Can you work these out from the model? Positions are in its coordinate system, mm. A direction names the side the tool comes from. Round coordinates to 2 decimals unless told otherwise and drop trailing zeros. Order: outer loops, then holes, each group sorted by start corner. A loop starts at its lowest first (then second) coordinate and runs counter-clockwise, first axis right, second up. Notation, with made-up numbers: (74.25, 66) -> (93.25, 66) arc R23 cw to (93.25, 80) -> close; hole circle Ø3 at (7.5, 60.25). An arc over 180 degrees is marked (long way). One line per item, written item: value.
Autodesk Inventor part; units mm, degrees
ref_plane "YZ Plane" through (0, 0, 0) normal (1, 0, 0) x (0, 1, 0)
ref_plane "XZ Plane" through (0, 0, 0) normal (0, 1, 0) x (-1, 0, 0)
ref_plane "XY Plane" through (0, 0, 0) normal (0, 0, 1) x (1, 0, 0)
sketch "Sketch1" plane through (0, 0, 0) normal (0, 1, 0) x (-1, 0, 0)
  line L0 (0, 0) -> (180.34, 0)
  line L1 (180.34, 0) -> (180.34, -76.2)
  line L2 (180.34, -76.2) -> (0, -76.2)
  line L3 (0, -76.2) -> (0, 0)
  dimension "d0" = 180.34
  dimension "d1" = 76.2
extrude "Extrusion1" add sketch "Sketch1" along normal blind 167.64
fillet "Fillet1" radius 3.175 8 edges at (-90.17, 167.64, 0) (-180.34, 167.64, -38.1) (-90.17, 167.64, -76.2) (0, 167.64, -38.1) (-90.17, 0, -76.2) (-180.34, 0, -38.1) (-90.17, 0, 0) (0, 0, -38.1)
sketch "Sketch2" plane through (0, 3.175, -76.2) normal (1, 0, 0) x (0, 0, -1)
  line L0 (0, 164.465) -> (-19.05, 164.465)
  line L1 (-19.05, 164.465) -> (-19.05, 145.415)
  line L2 (-19.05, 145.415) -> (0, 145.415)
  line L3 (0, 145.415) -> (0, 164.465)
  line L4 (0, 164.465) -> (-19.05, 164.465)
  line L5 (-19.05, 164.465) -> (-19.05, 145.415)
  line L6 (-19.05, 145.415) -> (0, 145.415)
  line L7 (0, 145.415) -> (0, 164.465)
  point P0 (-76.2, -3.175)
  dimension "d5" = 19.05
  dimension "d6" = 19.05
extrude "Extrusion2" cut sketch "Sketch2" against normal blind 50.8
sketch "Sketch3" plane through (-180.34, 3.175, 0) normal (-1, 0, 0) x (0, 0, 1)
  line L0 (-76.2, 164.465) -> (-57.15, 164.465)
  line L1 (-57.15, 164.465) -> (-57.15, 145.415)
  line L2 (-57.15, 145.415) -> (-76.2, 145.415)
  line L3 (-76.2, 145.415) -> (-76.2, 164.465)
  point P0 (0, -3.175)
  dimension "d9" = 19.05
  dimension "d10" = 19.05
extrude "Extrusion3" cut sketch "Sketch3" against normal blind 50.8
fillet "Fillet2" radius 3.175 22 edges at (-154.94, 148.59, -57.15) (-129.54, 148.59, -66.675) (-129.54, 158.115, -57.15) (-179.4101, 166.7101, -57.15) (-180.34, 156.5275, -57.15) (-153.3525, 167.64, -57.15) (-129.54, 166.7101, -75.2701) (-129.54, 156.5275, -76.2) (-129.54, 167.64, -65.0875) (-154.94, 148.59, -76.2) (-180.34, 148.59, -66.675) (-25.4, 148.59, -76.2) (-50.8, 166.7101, -75.2701) (-50.8, 167.64, -65.0875) (-50.8, 156.5275, -76.2) (-0.9299, 166.7101, -57.15) (0, 156.5275, -57.15) (-26.9875, 167.64, -57.15) (0, 148.59, -66.675) (-25.4, 148.59, -57.15) (-50.8, 148.59, -66.675) (-50.8, 158.115, -57.15)
properties part number "FRC Battery"
Q1. I want a section at B-B on y = 156.5. List the corners of the cut face in (x, z) for me (3 decimals), plus the area to 3 significant figures.
Answers below:
outline: (-180.34, -53.975) arc R3.175 ccw to (-177.165, -57.15) -> (-132.715, -57.15) arc R3.175 cw to (-129.54, -60.325) -> (-129.54, -73.025) arc R3.175 ccw to (-126.365, -76.2) -> (-53.975, -76.2) arc R3.175 ccw to (-50.8, -73.025) -> (-50.8, -60.325) arc R3.175 cw to (-47.625, -57.15) -> (-3.175, -57.15) arc R3.175 ccw to (0, -53.975) -> (0, 0) -> (-180.34, 0) -> close
area: 11,800 mm^2
Q2. Please list where these lines run through material, in increasing order: line 1 along Y through (x, z) = (-19, -67); line 2 along Y through (x, z) = (-40.5, -55.5).
Answers below:
line 1: 0 to 148.59
line 2: 0 to 167.25
Q3. Will these pins go through, and if not, where does the flat tip stop? pin 1 Ø4 at (x, z) = (-152.5, -68) entering from +Y; pin 2 Ø6.5 at (y, z) = (158, -68.5) entering from +X; pin 3 Ø14 at (y, z) = (160, -64.5) entering from -X.
Answers below:
pin 1: y = 148.59
pin 2: x = -50.8
pin 3: x = -131.27
Q4. I want a section at A-A on x = -147. List the corners of the cut face in (y, z) for me (3 decimals), plus the area to 3 significant figures.
Answers below:
outline: (0, -73.025) arc R3.175 ccw to (3.175, -76.2) -> (145.415, -76.2) arc R3.175 ccw to (148.59, -73.025) -> (148.59, -60.325) arc R3.175 cw to (151.765, -57.15) -> (164.465, -57.15) arc R3.175 ccw to (167.64, -53.975) -> (167.64, -3.175) arc R3.175 ccw to (164.465, 0) -> (3.175, 0) arc R3.175 ccw to (0, -3.175) -> close
area: 12,400 mm^2
Q5. On a 3-axis mill with a long thin cutter (end or side, diameter ignored), from which of +Z, -Z, +X, -X, +Y, -Y can I reach the whole of each face in a straight line? I mean faces 1 (the face through (-129.54, 158, -67)), 2 (the face through (-50.8, 158, -67)), 3 (the face through (0, 83, -39)). Say none if no direction works.
Answers below:
face 1: -Z, -X, +Y
face 2: -Z, +X, +Y
face 3: +Z, -Z, +X, +Y, -Y
